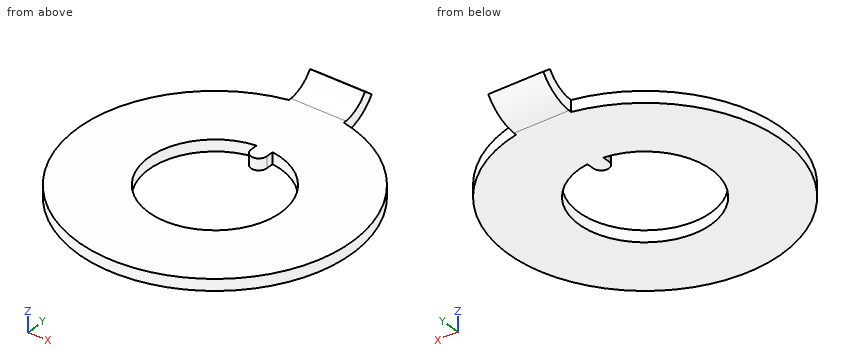
from build123d import *

# Parameters (mm, degrees)
SKETCH1_R           = 6
BOSS_EXTRUDE1_DEPTH = 0.5
BOSS_EXTRUDE2_START = -0.121225
SKETCH2_W           = 2.4
SKETCH2_H           = 0.5
BOSS_EXTRUDE2_DEPTH = 0.121225
SWEEP1_START        = -1.2
SWEEP1_DEPTH        = 2.4


# Read off the part's stored shape, not the designer's step: Sweep1
with BuildPart() as part:
    # Sketch1 → Boss-Extrude1 (new body)
    with BuildSketch(Plane.XY):
        Circle(SKETCH1_R)
        with BuildLine():
            Line((-0.35, 2.878801834), (-0.35, 2.55))
            ThreePointArc((-0.35, 2.55), (0, 2.2), (0.35, 2.55))
            Line((0.35, 2.55), (0.35, 2.878801834))
            ThreePointArc((0.35, 2.878801834), (0, -2.9), (-0.35, 2.878801834))
        make_face(mode=Mode.SUBTRACT)
    extrude(amount=BOSS_EXTRUDE1_DEPTH)

    # Sketch2 → Boss-Extrude2 (add)
    with BuildSketch(Plane(origin=(0, 6, 0), x_dir=(1, 0, 0), z_dir=(0, 1, 0)).offset(BOSS_EXTRUDE2_START)):
        with Locations((0, -0.25)):
            Rectangle(SKETCH2_W, SKETCH2_H)
    extrude(amount=BOSS_EXTRUDE2_DEPTH)

    # Sweep1 outline → Sweep1 (add)
    with BuildSketch(Plane.YZ.offset(SWEEP1_START)):
        with BuildLine():
            ThreePointArc((6, 0), (6.842994327, 0.249762545), (7.492047788, 0.84284801))
            Line((7.492047788, 0.84284801), (7.098940121, 1.151824324))
            ThreePointArc((7.098940121, 1.151824324), (6.624463044, 0.699478098), (6, 0.5))
            Line((6, 0.5), (6, 0))
        make_face()
    extrude(amount=SWEEP1_DEPTH)


solid = part.part
Geometry: final body of the model. Coordinates: model frame, mm. Round coordinates to 2 decimals unless told otherwise and drop trailing zeros. Loops run counter-clockwise (first coordinate to the right, second up) from the corner with the lowest first, then second, coordinate; pieces in that order, holes last. Notation, with made-up numbers: (71, -22) - (87, -22) arc R26 cw to (87, -3) - close; hole circle Ø3 at (-20, 24). An arc over 180 degrees is marked (long way). Write each question's results on one line, items separated by ' | '. Start each with the question number.
1) Cut plane D-D on x = -2.25. Return loops of the section in (y, z).
2) First-contact query: P1, Ø2, axis at x = -1, y = -0.5, coming from the -Z side. Flat tip, straight axial feed; report the tip coordinate or a pass-through.
3) Line query: probe 1 along X at (y, z) = (0, 0.3); probe 2 along Z at (x, y) = (-5, -3); probe 3 along Y at (x, z) = (-0.5, 0.25). Output: solid intervals per line, ascending. Write a range as [from, to].
4) Cut plane A-A on y = 0. Return loops of the section in (x, z), then the cut area to 3 significant figures.
5) Cut plane C-C on z = 0.15. Return loops of the section in (x, y), then the cut area to 3 significant figures.
6) Cut plane B-B on x = 0. Return loops of the section in (y, z), then the cut area to 3 significant figures.
Verdict:
1) outline: (-5.56, 0) - (-1.83, 0) - (-1.83, 0.5) - (-5.56, 0.5) - close; (1.83, 0) - (5.56, 0) - (5.56, 0.5) - (1.83, 0.5) - close
2) P1: passes through
3) probe 1: x = [-6, -2.9], [2.9, 6] | probe 2: z = [0, 0.5] | probe 3: y = [-5.98, -2.86], [2.86, 6.84]
4) outline: (-6, 0) - (-2.9, 0) - (-2.9, 0.5) - (-6, 0.5) - close; (2.9, 0) - (6, 0) - (6, 0.5) - (2.9, 0.5) - close | area: 3.10 mm2
5) outline: (-1.2, 5.88) arc R6 ccw (long way) to (1.2, 5.88) - (1.2, 6.64) - (-1.2, 6.64) - close; hole (-0.35, 2.55) - (-0.35, 2.88) arc R2.9 ccw (long way) to (0.35, 2.88) - (0.35, 2.55) arc R0.35 cw to start | area: 88.7 mm2
6) outline: (-6, 0) - (-2.9, 0) - (-2.9, 0.5) - (-6, 0.5) - close; (2.2, 0) - (6, 0) arc R1.96 ccw to (7.49, 0.84) - (7.1, 1.15) arc R1.46 cw to (6, 0.5) - (2.2, 0.5) - close | area: 4.22 mm2
